Check sheet for the drawn part. Datum: minimum x, y, z corner. Units: mm. A direction names the side the tool comes from. Give positions to 0.01 mm unless a question says otherwise; leave off trailing zeros. Write each loop counter-clockwise with the first axis right and the second up, starting at its lowest first coordinate (ties: lowest second). Pieces come first, ordered by that corner, then holes. Notation, with made-up numbers: (-30.5, -27.75) - (22.5, -27.75) arc R17 ccw to (22.5, -1.75) - close; hole circle Ø9 at (-34, 35.5). An arc over 180 degrees is marked (long way). One line per question, with ' | ' between items. Start each with the question number.
Q1. Set-up check for the marked faces 1, 2, 3 and 4: record each of +Z, -Z, +X, -X, +Y, -Y from which the full face is reachable in a straight line by a thin tool's end or side.
Q2. Gauge pin test, flat ends, axial feed: P1, Ø5.5, axis at x = 18, y = 63.5, coming from the +Z side; P2, Ø1, axis at y = 144.5, z = 43.5, coming from the +X side (1 decimal); P3, Ø3, axis at x = 32.5, z = 12, coming from the -Y side (1 decimal). Record the tip position at first contact, or that the pin passes through.
Q3. Section check A-A on y = 12. Record the boundary of the cut face in (x, z) (1 decimal).
Q4. Thickness scan on L1, parallel to Y at x = 37, z = 26.5; L2, parallel to Y at x = 46, z = 18; L3, parallel to Z at x = 37, y = 71 (1 decimal). Record the ranges inside material, lowest first. Write a range as [from, to].
Q5. Section check B-B on y = 162.5. Record the boundary of the cut face in (x, z) (1 decimal), and give its area (3 significant figures).
Q6. Release check for a two-part mould opening along Y. For the marked faces 5, 6, 7 and 8 record: +Y half, -Y half, draft (parallel to the pull), parting line (faces both ways), or undercut.
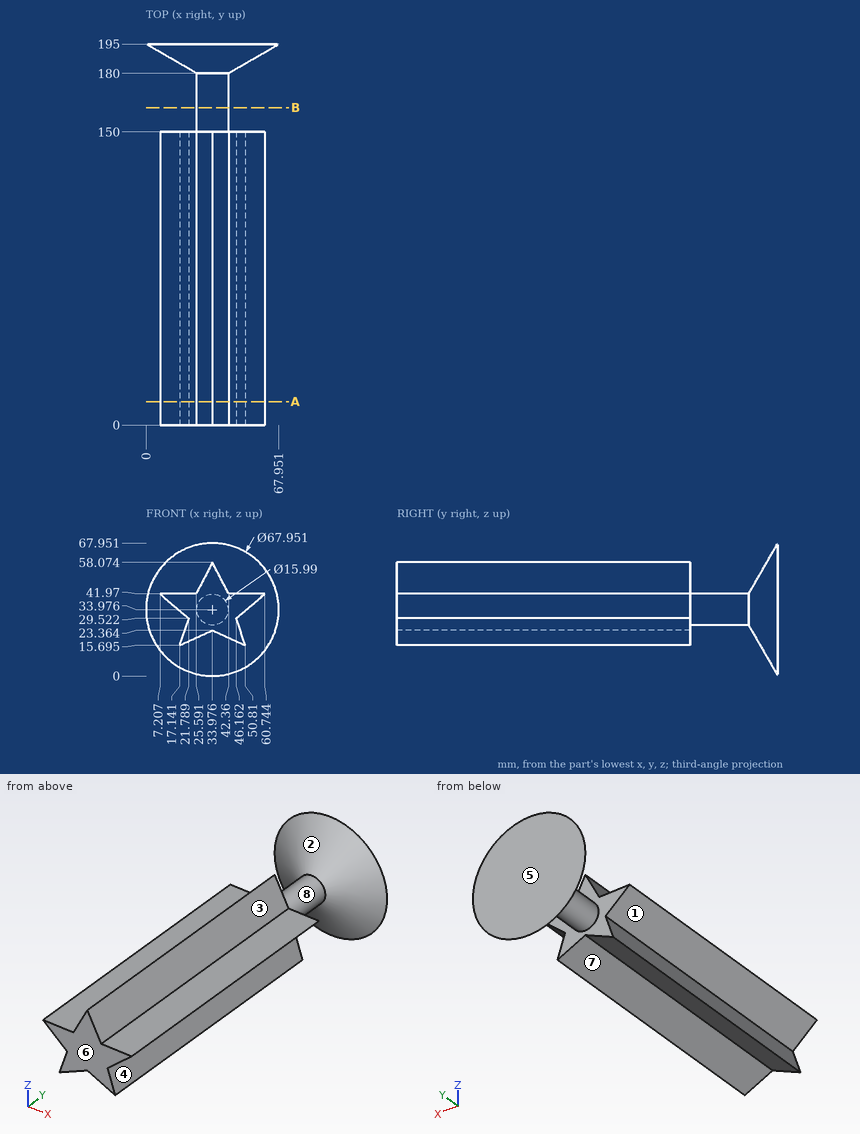
Working result:
1) face 1: -X, -Y | face 2: none | face 3: +Z, +X, -Y | face 4: +X, -Y
2) P1: stops at z = 41.97 | P2: stops at x = 41.8 | P3: stops at y = 187.2
3) outline: (7.2, 42) - (21.8, 29.5) - (17.1, 15.7) - (34, 23.4) - (50.8, 15.7) - (46.2, 29.5) - (60.7, 42) - (42.4, 42) - (34, 58.1) - (25.6, 42) - close
4) L1: y = [0, 150], [180.04, 195] | L2: y = [0, 150], [186.93, 195] | L3: z = [22, 52.3]
5) outline: circle Ø16 at (34, 34) | area: 201 mm2
6) face 5: +Y half | face 6: -Y half | face 7: draft | face 8: undercut
